Read the model definition and answer for the solid it produces. Units are mm, in the model's axes. Face numbers are marked on the shaded views. A direction names the side the tool comes from. Coordinates: 2 decimals unless noted, no trailing zeros. Write each loop counter-clockwise with the first axis right and the second up, starting at its lowest first coordinate (ties: lowest second). Pieces come first, ordered by that corner, then holes.
1) The part is cut by section B-B (z = 5). Determine the outline of the cut face in (x, y).
2) Each of these flat-tipped pins is pushed along its axis until it touches: pin 1 Ø6.5 at (y, z) = (-0.5, 37) entering from +X; pin 2 Ø1.5 at (x, z) = (29, 38) entering from +Y; pin 3 Ø2 at (y, z) = (-8.5, 9.5) entering from -X; pin 4 Ø8 at (x, z) = (-6, 8) entering from +Y. Where does it stop, or does it pass through?
3) The part is cut by section C-C (z = 45). Determine the outline of the cut face in (x, y) (3 decimals).
4) Find the intervals of material crossed by line 1 (Z direction, x = -10.35, y = 0); line 2 (Y direction, x = -17.55, z = 45); line 3 (Z direction, x = -32.5, y = 13), in increasing order.
5) Which of the six approach directions +Z, -Z, +X, -X, +Y, -Y give full straight-line access (tool end or side, diameter ignored) to the marked faces 1, 2, 3 and 4?
6) The part is cut by section A-A (z = 31). Determine the outline of the cut face in (x, y), then the cut area to 3 significant figures.
7) Determine the mould class of the marked faces 5, 6, 7 and 8 for opening direction Y: +Y half, -Y half, draft (parallel to the pull), parting line (faces both ways), or undercut.
from build123d import *

# Parameters (mm, degrees)
F3_DEPTH = 50.001
F4_R     = 2.6
F5_DEPTH = 37.501
F9_DEPTH = 2.25
F10_R    = 2
F11_SIZE = 1


with BuildPart() as f1:
    # F0 (on Front) → F1 (revolve)
    with BuildSketch(Plane.XZ):
        Polygon((0, 0), (17.5, 0), (31.5, 35), (37.5, 35), (37.5, 40), (20, 40), (20, 50), (0, 50), align=None)
    revolve(axis=Axis((0, 0, 25), (0, 0, -1)))

    # F2 (on face) → F3 (cut, through all)
    with BuildSketch(Plane.XY.offset(50)):
        Polygon((0, -8.371579), (7.25, -4.185789), (7.25, 4.185789), (0, 8.371579), (-7.25, 4.185789), (-7.25, -4.185789), align=None)
    extrude(amount=-F3_DEPTH, mode=Mode.SUBTRACT)

    # F4 (on Right) → F5 (cut, through all)
    with BuildSketch(Plane.YZ):
        with Locations((0, 45)):
            Circle(F4_R)
    extrude(amount=-F5_DEPTH, mode=Mode.SUBTRACT)

    # F8 (on face) → F9 (cut, symmetric)
    with BuildSketch(Plane.YZ.offset(-13.625)):
        Polygon((4.1, 42.632864), (4.1, 55), (-4.1, 55), (-4.1, 42.632864), (0, 40.265728), align=None)
    extrude(amount=F9_DEPTH, both=True, mode=Mode.SUBTRACT)

    # F10
    f10_edges = [f1.edges().sort_by_distance(p)[0] for p in [
        (-20, 0, 50),
        (-20, 0, 40),
        (-37.5, 0, 40),
        (-37.5, 0, 35),
        (-17.5, 0, 0),
        (-3.625, -6.278684, 0),
        (3.625, -6.278684, 0),
        (7.25, 0, 0),
        (3.625, 6.278684, 0),
        (-3.625, 6.278684, 0),
        (-7.25, 0, 0),
    ]]
    fillet(f10_edges, radius=F10_R)

    # F11
    f11_edges = [f1.edges().sort_by_distance(p)[0] for p in [
        (-13.625, 4.1, 50),
        (-11.375, 0, 50),
        (-13.625, -4.1, 50),
        (-15.875, 0, 50),
    ]]
    chamfer(f11_edges, length=F11_SIZE)


solid = f1.part
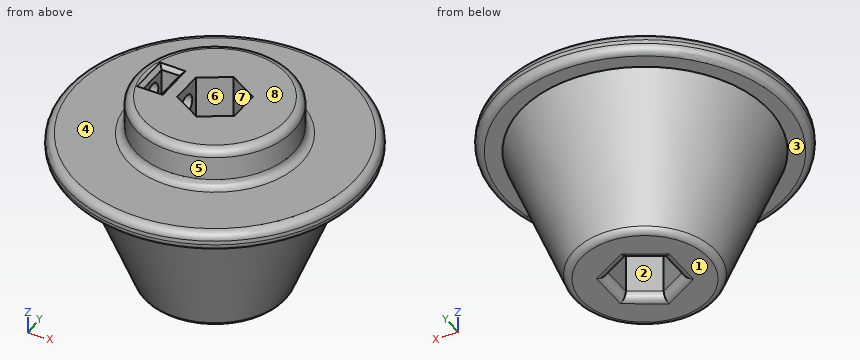
Reported:
1. outline: circle Ø39 at (0, 0); hole (-7.25, -4.19) - (0, -8.37) - (7.25, -4.19) - (7.25, 4.19) - (0, 8.37) - (-7.25, 4.19) - close
2. pin 1: stops at x = 37.5
2. pin 2: stops at y = 24.66
2. pin 3: stops at x = -20.13
2. pin 4: stops at y = 21.73
3. outline: (-19.83, -2.6) arc R20 ccw (long way) to (-19.83, 2.6) - (-15.875, 2.6) - (-15.875, 4.1) - (-11.375, 4.1) - (-11.375, 2.6) - (-7.25, 2.6) - (-7.25, 4.186) - (0, 8.372) - (7.25, 4.186) - (7.25, -4.186) - (0, -8.372) - (-7.25, -4.186) - (-7.25, -2.6) - (-11.375, -2.6) - (-11.375, -4.1) - (-15.875, -4.1) - (-15.875, -2.6) - close
4. line 1: z = 0 to 42.4, 47.6 to 50
4. line 2: y = -9.59 to -2.6, 2.6 to 9.59
4. line 3: z = 35 to 40
5. face 1: -Z, +X, -X, +Y, -Y
5. face 2: +Z, -Z
5. face 3: -Z
5. face 4: +Z
6. outline: circle Ø59.8 at (0, 0); hole (-7.25, -4.19) - (0, -8.37) - (7.25, -4.19) - (7.25, 4.19) - (0, 8.37) - (-7.25, 4.19) - close
6. area: 2,630 mm2
7. face 5: parting line
7. face 6: undercut
7. face 7: undercut
7. face 8: draft
